Check sheet for the modelled part. Datum: model origin and axes. Units: mm. Face numbers are marked on the shaded views. A direction names the side the tool comes from. Give positions to 0.01 mm unless a question says otherwise; leave off trailing zeros. Loops run counter-clockwise (first coordinate to the right, second up) from the corner with the lowest first, then second, coordinate; pieces in that order, holes last. Notation, with made-up numbers: (-27, -7.75) - (10, -7.75) arc R33 ccw to (10, 29.25) - close; hole circle Ø11 at (54.25, -28.5). An arc over 180 degrees is marked (long way). Answer in a Markdown table with one row per item. Add a question column.
(1) Go/stop test with flat-tipped pins: P1, Ø3, axis at y = -12.5, z = 0.5, coming from the -X side; P2, Ø10, axis at y = -0.5, z = -10.5, coming from the -X side; P3, Ø12, axis at x = -18, y = -11, coming from the -Z side; P4, Ø3, axis at y = -27.5, z = -10, coming from the -X side. Record where each tip stops, or that it passes through.
(2) Sectioned sample at A-A on y = -32. Enter the section's corners in (x, z).
(3) Set-up check for the marked faces 1 and 2: record each of +Z, -Z, +X, -X, +Y, -Y from which the full face is reachable in a straight line by a thin tool's end or side.
(4) Thickness scan on L1, parallel to Z at x = -10, y = -12; L2, parallel to Y at x = -15.25, z = -13; L3, parallel to X at y = -12.5, z = -8.5. Record the ranges inside material, lowest first.
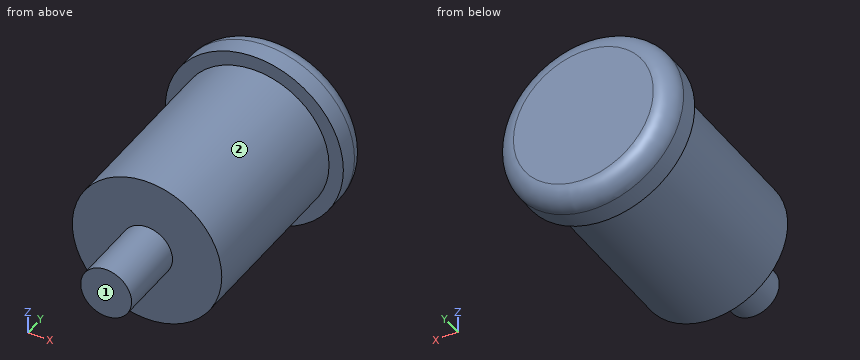
from build123d import *

# Parameters (mm, degrees)
SKETCH1_R           = 14
BOSS_EXTRUDE1_DEPTH = 6
SKETCH2_R           = 11.75
BOSS_EXTRUDE2_DEPTH = 28.85
FILLET1_R           = 3
SKETCH3_R           = 4
BOSS_EXTRUDE3_DEPTH = 11


with BuildPart() as part:
    # Sketch1 → Boss-Extrude1 (new body)
    with BuildSketch(Plane(origin=(0, 0, 0), x_dir=(1, 0, 0), z_dir=(0, 1, 0))):
        with Locations((-10.425597089, 8.327180584)):
            Circle(SKETCH1_R)
    extrude(amount=BOSS_EXTRUDE1_DEPTH)

    # Sketch2 → Boss-Extrude2 (add)
    with BuildSketch(Plane.XZ):
        with Locations((-10.425597089, -8.327180584)):
            Circle(SKETCH2_R)
    extrude(amount=BOSS_EXTRUDE2_DEPTH)

    # Fillet1
    fillet1_edges = [part.edges().sort_by_distance(p)[0] for p in [
        (-24.425597089, 6, -8.327180584),
    ]]
    fillet(fillet1_edges, radius=FILLET1_R)

    # Sketch3 → Boss-Extrude3 (add)
    with BuildSketch(Plane.XZ.offset(28.85)):
        with Locations((-10.425597089, -8.327180584)):
            Circle(SKETCH3_R)
    extrude(amount=BOSS_EXTRUDE3_DEPTH)


solid = part.part
Reply:
| question | item | result |
|---|---|---|
| 1 | P1 | x = -19.61 |
| 1 | P2 | x = -24.43 |
| 1 | P3 | z = -19.97 |
| 1 | P4 | x = -22.17 |
| 2 | outline | circle Ø8 at (-10.43, -8.33) |
| 3 | face 1 | +Z, -Z, +X, -X, -Y |
| 3 | face 2 | -Y |
| 4 | L1 | -20.07 to 3.42 |
| 4 | L2 | -28.85 to 6 |
| 4 | L3 | -22.17 to 1.32 |
